from build123d import *

# Parameters (mm, degrees)
SKETCH4_R           = 10.429730926
SKETCH4_R_2         = 7.9
CUT_EXTRUDE1_DEPTH  = 0.5
SKETCH5_R           = 6.75
CUT_EXTRUDE2_DEPTH  = 0.5
SKETCH6_R           = 4.25
BOSS_EXTRUDE1_DEPTH = 0.5
SKETCH7_R           = 2.5
CUT_EXTRUDE3_DEPTH  = 21.372315774


with BuildPart() as part:
    # Sketch1 → Revolve1 (revolve)
    with BuildSketch(Plane.XY, mode=Mode.PRIVATE) as revolve1_sk:
        Polygon((0, 0), (-8.999444444, 0), (-12.125, 2.5), (-12.125, 8.5), (-8.999444444, 11), (0, 11), align=None)
    revolve(revolve1_sk.sketch.rotate(Axis((0, 11, 0), (0, -1, 0)), 270), axis=Axis((0, 11, 0), (0, -1, 0)))

    # Sketch4 → Cut-Extrude1 (cut)
    with BuildSketch(Plane(origin=(0, 11, 0), x_dir=(1, 0, 0), z_dir=(0, 1, 0))):
        Circle(SKETCH4_R)
        with Locations(Location((0, 0, 0), (0, 0, 270))):
            Circle(SKETCH4_R_2, mode=Mode.SUBTRACT)
    cut_extrude1 = extrude(amount=-CUT_EXTRUDE1_DEPTH, mode=Mode.SUBTRACT)

    # Sketch5 → Cut-Extrude2 (cut)
    with BuildSketch(Plane(origin=(0, 11, 0), x_dir=(1, 0, 0), z_dir=(0, 1, 0))):
        with Locations(Location((0, 0, 0), (0, 0, 270))):
            Circle(SKETCH5_R)
    cut_extrude2 = extrude(amount=-CUT_EXTRUDE2_DEPTH, mode=Mode.SUBTRACT)

    # Sketch6 → Boss-Extrude1 (add)
    with BuildSketch(Plane(origin=(0, 10.5, 0), x_dir=(1, 0, 0), z_dir=(0, 1, 0))):
        with Locations(Location((0, 0, 0), (0, 0, 270))):
            Circle(SKETCH6_R)
    boss_extrude1 = extrude(amount=BOSS_EXTRUDE1_DEPTH)

    # Mirror1: Cut-Extrude1, Cut-Extrude2, Boss-Extrude1 across plane
    add(cut_extrude1.mirror(Plane.ZX.offset(5.5)), mode=Mode.SUBTRACT)
    add(cut_extrude2.mirror(Plane.ZX.offset(5.5)), mode=Mode.SUBTRACT)
    add(boss_extrude1.mirror(Plane.ZX.offset(5.5)))

    # Sketch7 → Cut-Extrude3 (cut, through all)
    with BuildSketch(Plane(origin=(0, 11, 0), x_dir=(1, 0, 0), z_dir=(0, 1, 0))):
        with Locations(Location((0, 0, 0), (0, 0, 270))):
            Circle(SKETCH7_R)
    extrude(amount=-CUT_EXTRUDE3_DEPTH, mode=Mode.SUBTRACT)


solid = part.part
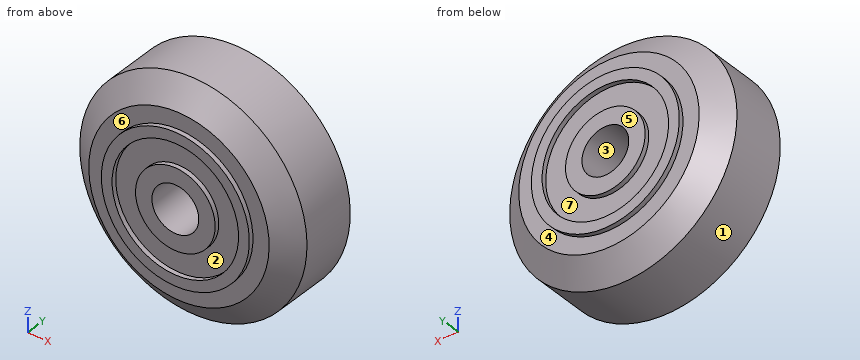
CAD build for the part. Positions are in the model's coordinates, mm. Face numbers are marked on the shaded views. A direction names the side the tool comes from. Round coordinates to 2 decimals unless told otherwise and drop trailing zeros. Loops run counter-clockwise (first coordinate to the right, second up) from the corner with the lowest first, then second, coordinate; pieces in that order, holes last. Notation, with made-up numbers: (1.5, 57) - (20.5, 57) arc R20 cw to (20.5, 75) - close; hole circle Ø7 at (-21, -37). An arc over 180 degrees is marked (long way). Put each result on its own line as item: value.
1. 3-axis set-ups, long thin cutter, end or side, ignore diameter. For the marked faces 5, 6 and 7: which of +Z, -Z, +X, -X, +Y, -Y reach the whole face in a straight line?
Geometry check:
face 5: +Z, -Z, +X, -X, +Y
face 6: -Y
face 7: +Y
2. Slice it at A-A on y = 3. List the corners of the cut face in (x, z) (3 decimals).
Geometry check:
outline: circle Ø24.25 at (0, 0); hole circle Ø5 at (0, 0)
3. Wall check: line 1 (X direction, y = 10.7, z = 0); line 2 (X direction, y = 6, z = 0) (3 decimals); line 3 (Y direction, x = 0, z = 9.5). Give the ranges that are in metal, low to high.
Geometry check:
line 1: -7.9 to -6.75, -4.25 to -2.5, 2.5 to 4.25, 6.75 to 7.9
line 2: -12.125 to -2.5, 2.5 to 12.125
line 3: 0.5 to 10.5
4. Pin check, flat tips, straight feed: P1, Ø2, axis at x = 2.5, y = 5, coming from the -Z side; P2, Ø4, axis at y = 7.5, z = -8, coming from the +X side; P3, Ø6, axis at x = 7, z = 5, coming from the -Y side; P4, Ø1, axis at x = 8, z = -6, coming from the -Y side. Stop position of each tip, or through.
Geometry check:
P1: z = -12.03
P2: x = 10.54
P3: y = 0
P4: y = 0.5
5. Two-plate mould, pull along Z, no slides. Class the marked faces 1, 2, 3 and 4: released by +Z, released by -Z, zero draft, split by the parting line, or undercut.
Geometry check:
face 1: split by the parting line
face 2: undercut
face 3: undercut
face 4: zero draft
